Source: CAD feature listing. Evaluate the final solid. Frame: model axes, mm. A direction names the side the tool comes from. Coordinates: 2 decimals unless noted, no trailing zeros. Order: outer loops, then holes, each group sorted by start corner. A loop starts at its lowest first (then second) coordinate and runs counter-clockwise, first axis right, second up.
Item 1: Section B-B on z = 12.5. Return the cut outline in (x, y), then the cut area to 3 significant figures.
Item 2: Reachability of faces 1 (the flat face through (-11.19, 45.48, 64.88)), 2 (the flat face through (-47, 3.968, -48)), 3 (the flat face through (0, 44, -10.927)), 4 (the flat face through (-59.279, 45.479, -18.423)) from +Z, -Z, +X, -X, +Y, -Y: full face, straight path, thin tool, end or side. Return the list, or none.
Item 3: Mould query, pull axis X, two halves, no side actions, for faces 5 (the flat face through (13.69, 45.48, 60.55)), 6 (the cylindrical face through (-3.367, 45.166, -0.748)), 7 (the cylindrical face through (75, 45.48, -13.38)), 8 (the flat face through (-31.7, 45.5, 59.4)). Classes: released by +X, released by -X, zero draft, split by the parting line, or undercut.
Item 4: Contact query for flat-ended pins moving along their axis: P1, Ø1.5, axis at y = 10, z = 9.5, coming from the +X side; P2, Ø21.5, axis at x = 61, z = -18, coming from the -Y side; P3, Ø11, axis at y = 92, z = -47.5, coming from the -X side. Output: stop coordinate, or through.
Item 5: Section C-C on x = 53.5. Return the cut outline in (y, z), then the cut area to 3 significant figures.
Item 6: Section A-A on x = 26.5. Return the cut outline in (y, z).
Item 7: Ray query, line 1 (X direction, y = 89.5, z = -53); line 2 (X direction, y = 51, z = 65); line 3 (Z direction, x = 36, y = 1.5). Return the intervals inside material, ascending.
from build123d import *

# Parameters (mm, degrees)
SALIENTE_EXTRUIR1_DEPTH = 88.9
CROQUIS4_R              = 2.999994
CORTAR_EXTRUIR1_DEPTH   = 112.44204772
REDONDEO6_R             = 3
REDONDEO7_R             = 3
ESCALA2_SCALE           = 1.15
SALIENTE_EXTRUIR3_DEPTH = 101.6
CROQUIS10_W             = 32
CROQUIS10_H             = 81.6
CORTAR_EXTRUIR2_DEPTH   = 15


with BuildPart() as part:
    # Croquis1 → Saliente-Extruir1 (new body)
    with BuildSketch(Plane(origin=(0, 0, 0), x_dir=(1, 0, 0), z_dir=(0, 1, 0))):
        Polygon((1.696358741, -16.064461222), (13.335, -27.703102481), (0, -50.8), (-13.335, -27.703102481), (-1.696358741, -16.064461222), (-14.760410887, 6.563140847), (-30.659090512, 2.303102481), (-43.994090512, 25.4), (-17.324090512, 25.4), (-13.064052146, 9.501320374), (13.064052146, 9.501320374), (17.324090512, 25.4), (43.994090512, 25.4), (30.659090512, 2.303102481), (14.760410887, 6.563140847), align=None)
    extrude(amount=SALIENTE_EXTRUIR1_DEPTH)

    # Croquis4 → Cortar-Extruir1 (cut, through all)
    with BuildSketch(Plane(origin=(0, 88.9, 0), x_dir=(1, 0, 0), z_dir=(0, 1, 0))):
        with Locations(Location((0, 0, 0), (0, 0, 270))):
            Circle(CROQUIS4_R)
    extrude(amount=-CORTAR_EXTRUIR1_DEPTH, mode=Mode.SUBTRACT)

    # Redondeo6
    redondeo6_edges = [part.edges().sort_by_distance(p)[0] for p in [
        (-1.696358741, 44.45, 16.064461222),
        (-14.760410887, 44.45, -6.563140847),
        (-13.064052146, 44.45, -9.501320374),
        (13.064052146, 44.45, -9.501320374),
        (1.696358741, 44.45, 16.064461222),
    ]]
    fillet(redondeo6_edges, radius=REDONDEO6_R)

    # Redondeo7
    redondeo7_edges = [part.edges().sort_by_distance(p)[0] for p in [
        (-13.335, 44.45, 27.703102481),
        (-30.659090512, 44.45, -2.303102481),
        (-17.324090512, 44.45, -25.4),
        (17.324090512, 44.45, -25.4),
        (30.659090512, 44.45, -2.303102481),
        (13.335, 44.45, 27.703102481),
    ]]
    fillet(redondeo7_edges, radius=REDONDEO7_R)


with BuildPart() as part_1:
    # Escala2: scaled about (-0.008124988, 44.45, 0.003254237)
    add(part.part.scale(ESCALA2_SCALE).moved(Location((0.001218748, -6.6675, -0.000488136))))

    # Croquis8 → Saliente-Extruir3 (add)
    with BuildSketch(Plane(origin=(0, 95.5675, 0), x_dir=(1, 0, 0), z_dir=(0, 1, 0))):
        with BuildLine():
            Line((-50.591985341, 54.687778623), (-50.591985341, 29.210488136))
            Line((-50.591985341, 29.210488136), (-45.591985341, 29.210488136))
            Line((-45.591985341, 29.210488136), (-45.591985341, 54.687778623))
            Line((-45.591985341, 54.687778623), (-35.591985341, 54.687778623))
            Line((-35.591985341, 54.687778623), (-35.591985341, 59.687778623))
            Line((-35.591985341, 59.687778623), (-45.591985341, 59.687778623))
            ThreePointArc((-45.591985341, 59.687778623), (-49.127519247, 58.223312529), (-50.591985341, 54.687778623))
        make_face()
        with BuildLine():
            Line((-48.092688033, 24.881578215), (-50.591985341, 29.210488136))
            Line((-50.591985341, 29.210488136), (-50.592688033, 29.211705234))
            Line((-50.592688033, 29.211705234), (-72.656668815, 16.47305999))
            ThreePointArc((-72.656668815, 16.47305999), (-74.228672243, 15.044447763), (-75.065739696, 13.092155328))
            ThreePointArc((-75.065739696, 13.092155328), (-75.082537721, 12.995468496), (-75.099211211, 12.89876011))
            ThreePointArc((-75.099211211, 12.89876011), (-75.070496458, 11.218650606), (-74.486795834, 9.642932971))
            Line((-74.486795834, 9.642932971), (-69.486795834, 0.982678934))
            Line((-69.486795834, 0.982678934), (-65.156668815, 3.482678934))
            Line((-65.156668815, 3.482678934), (-70.156668815, 12.142932971))
            Line((-70.156668815, 12.142932971), (-48.092688033, 24.881578215))
        make_face()
        with BuildLine():
            Line((72.656998235, 16.471842892), (50.593017453, 29.210488136))
            Line((50.593017453, 29.210488136), (48.093017453, 24.880361117))
            Line((48.093017453, 24.880361117), (70.156998235, 12.141715873))
            Line((70.156998235, 12.141715873), (65.156998235, 3.481461835))
            Line((65.156998235, 3.481461835), (69.487125254, 0.981461835))
            Line((69.487125254, 0.981461835), (74.487125254, 9.641715873))
            ThreePointArc((74.487125254, 9.641715873), (74.986627366, 13.435811098), (72.656998235, 16.471842892))
        make_face()
        with BuildLine():
            ThreePointArc((50.594422837, 54.687778623), (49.129956743, 58.223312529), (45.594422837, 59.687778623))
            Line((45.594422837, 59.687778623), (35.594422837, 59.687778623))
            Line((35.594422837, 59.687778623), (35.594422837, 54.687778623))
            Line((35.594422837, 54.687778623), (45.594422837, 54.687778623))
            Line((45.594422837, 54.687778623), (45.594422837, 29.210488136))
            Line((45.594422837, 29.210488136), (50.593017453, 29.210488136))
            Line((50.593017453, 29.210488136), (50.594422837, 29.210488136))
            Line((50.594422837, 29.210488136), (50.594422837, 54.687778623))
        make_face()
        with BuildLine():
            Line((2.499813364, -54.089384846), (0.000516056, -58.418294766))
            Line((0.000516056, -58.418294766), (-0.000186636, -58.419511864))
            Line((-0.000186636, -58.419511864), (22.063794146, -71.158157108))
            ThreePointArc((22.063794146, -71.158157108), (25.857889371, -71.657659221), (28.893921165, -69.328030089))
            Line((28.893921165, -69.328030089), (33.893921165, -60.667776052))
            Line((33.893921165, -60.667776052), (29.563794146, -58.167776052))
            Line((29.563794146, -58.167776052), (24.563794146, -66.828030089))
            Line((24.563794146, -66.828030089), (2.499813364, -54.089384846))
        make_face()
        with BuildLine():
            Line((-22.063464726, -71.15694001), (0.000516056, -58.418294766))
            Line((0.000516056, -58.418294766), (-2.499483944, -54.088167747))
            Line((-2.499483944, -54.088167747), (-24.563464726, -66.826812991))
            Line((-24.563464726, -66.826812991), (-29.563464726, -58.166558953))
            Line((-29.563464726, -58.166558953), (-33.893591745, -60.666558953))
            Line((-33.893591745, -60.666558953), (-28.893591745, -69.326812991))
            ThreePointArc((-28.893591745, -69.326812991), (-25.857559952, -71.656442122), (-22.063464726, -71.15694001))
        make_face()
    extrude(amount=-SALIENTE_EXTRUIR3_DEPTH)

    # Croquis10 → Cortar-Extruir2 (cut)
    with BuildSketch(Plane.ZY.offset(50.591985341)):
        with Locations((-45.210488136, 44.7675)):
            Rectangle(CROQUIS10_W, CROQUIS10_H)
    extrude(amount=-CORTAR_EXTRUIR2_DEPTH, mode=Mode.SUBTRACT)


solid = part_1.part
Answer list:
1. outline: (-5.4, -6.67) - (5.4, -6.67) - (5.4, 95.57) - (-5.4, 95.57) - close
1. area: 1,100 mm2
2. face 1: +Z, +Y, -Y
2. face 2: -Z, -X
2. face 3: -Z, +Y, -Y
2. face 4: +Y, -Y
3. face 5: undercut
3. face 6: undercut
3. face 7: released by +X
3. face 8: released by -X
4. P1: stops at x = 7.57
4. P2: stops at y = -6.03
4. P3: stops at x = -50.59
5. outline: (-6.03, -27.53) - (95.57, -27.53) - (95.57, -21.76) - (-6.03, -21.76) - close
5. area: 587 mm2
6. outline: (-6.67, -29.21) - (95.57, -29.21) - (95.57, -5) - (-6.67, -5) - close; (-6.03, 63.47) - (95.57, 63.47) - (95.57, 71.44) - (-6.03, 71.44) - close
7. line 1: x = -50.59 to -45.59, 45.59 to 50.59
7. line 2: x = -31.39 to -25.62, -21.4 to -11.4, 11.4 to 21.4, 25.62 to 31.39
7. line 3: z = -59.69 to -54.69, -29.21 to -4.19
